Design review of the part built by this model. Coordinates are the model's own, in mm. A direction names the side the tool comes from. Coordinates: 2 decimals unless noted, no trailing zeros. Loops run counter-clockwise (first coordinate to the right, second up) from the corner with the lowest first, then second, coordinate; pieces in that order, holes last. Notation, with made-up numbers: M -9,2 L 33,2 A16 ccw 33,8 Z; hole C -31.5,68 d1. An arc over 180 degrees is marked long. One line per item, written item: value.
```python
from build123d import *

# Parameters (mm, degrees)
EXTRUDE_1_DEPTH     = 14
SKETCH_3_R          = 4.25
CUT_EXTRUDE_1_DEPTH = 51.5
SKETCH_4_R          = 8
CUT_EXTRUDE_2_DEPTH = 46


with BuildPart() as part:
    # 草图1 → 凸台-拉伸1 (new body, symmetric)
    with BuildSketch(Plane.XY):
        Polygon((-100.5, -42.991652571), (-79.5, -42.991652571), (-79.5, 0.008347429), (79.5, 0.008347429), (79.5, -42.991652571), (100.5, -42.991652571), (100.5, -23.151157314), (81.63217636, 7.508347429), (-81.63217636, 7.508347429), (-100.5, -23.151157314), align=None)
    extrude(amount=EXTRUDE_1_DEPTH, both=True)

    # 草图3 → 切除-拉伸1 (cut, through all)
    with BuildSketch(Plane.XZ.offset(42.991652571)):
        with Locations((-90, 0)):
            Circle(SKETCH_3_R)
        with Locations((90, 0)):
            Circle(SKETCH_3_R)
    extrude(amount=-CUT_EXTRUDE_1_DEPTH, mode=Mode.SUBTRACT)

    # 草图4 → 切除-拉伸2 (cut)
    with BuildSketch(Plane(origin=(0, 7.508347429, 0), x_dir=(1, 0, 0), z_dir=(0, 1, 0))):
        with Locations((-90, 0)):
            Circle(SKETCH_4_R)
        with Locations((90, 0)):
            Circle(SKETCH_4_R)
    extrude(amount=-CUT_EXTRUDE_2_DEPTH, mode=Mode.SUBTRACT)


solid = part.part
```
(1) We need section C-C on x = 90. State the section outline as (y, z) points.
Reply:
outline: M -42.99,-14 L -6.09,-14 L -6.09,-8 L -38.49,-8 L -38.49,-4.25 L -42.99,-4.25 Z; M -42.99,4.25 L -38.49,4.25 L -38.49,8 L -6.09,8 L -6.09,14 L -42.99,14 Z
(2) We need section B-B on z = 0. State the section outline as (x, y) points.
Reply:
outline: M -100.5,-42.99 L -94.25,-42.99 L -94.25,-38.49 L -98,-38.49 L -98,-19.09 L -100.5,-23.15 Z; M -85.75,-42.99 L -79.5,-42.99 L -79.5,0.01 L 79.5,0.01 L 79.5,-42.99 L 85.75,-42.99 L 85.75,-38.49 L 82,-38.49 L 82,6.91 L 81.63,7.51 L -81.63,7.51 L -82,6.91 L -82,-38.49 L -85.75,-38.49 Z; M 94.25,-42.99 L 100.5,-42.99 L 100.5,-23.15 L 98,-19.09 L 98,-38.49 L 94.25,-38.49 Z
(3) Insertion check: pin 1 (7 mm diameter, centred on x = 90, z = 0, fed in from -Y); pin 2 (8.5 mm diameter, centred on x = -33.5, z = -5, fed in from -Y); pin 3 (13 mm diameter, centred on x = -89.5, z = -0.5, fed in from +Y); pin 4 (13 mm diameter, centred on x = 86, z = 1.5, fed in from +Y). Each pin has a flat end and moves straight along its axis. Give the tip position at first contact, or say it passes through.
Reply:
pin 1: passes through
pin 2: stops at y = 0.01
pin 3: stops at y = -38.49
pin 4: stops at y = 7.51
(4) We need section A-A on y = -16. State the section outline as (x, z) points.
Reply:
outline: M -96.1,-14 L -79.5,-14 L -79.5,14 L -96.1,14 L -96.1,5.18 A8 cw long -96.1,-5.18 Z; M 79.5,-14 L 96.1,-14 L 96.1,-5.18 A8 cw long 96.1,5.18 L 96.1,14 L 79.5,14 Z
(5) Mouldability with a two-part tool opening along Z and no side actions: class faces 4 (the flat face through (95.39, -14.85, 6.42)), 5 (the flat face through (7, 1, -14)), 6 (the cylindrical face through (85.754, -40.773, 0.187)), 7 (the cylindrical face through (-94.246, -40.773, 0.187)) as released by +Z, released by -Z, zero draft, split by the parting line, or undercut.
Reply:
face 4: zero draft
face 5: released by -Z
face 6: undercut
face 7: undercut
(6) We need section D-D on x = 61. State the section outline as (y, z) points, then the cut area to 3 significant figures.
Reply:
outline: M 0.01,-14 L 7.51,-14 L 7.51,14 L 0.01,14 Z
area: 210 mm2
(7) To check wall thickness, follow line 1 along X through (y, z) = (-26, 0); line 2 along X through (y, z) = (-24, -11.75); line 3 along X through (y, z) = (-26, -1.25). State the ranges of each line that lie inside material, in increasing order. Write a range as [from, to].
Reply:
line 1: x = [-100.5, -98], [-82, -79.5], [79.5, 82], [98, 100.5]
line 2: x = [-100.5, -79.5], [79.5, 100.5]
line 3: x = [-100.5, -97.9], [-82.1, -79.5], [79.5, 82.1], [97.9, 100.5]
(8) Tool access review of faces 1 (the flat face through (100.5, -33, 0)), 2 (the flat face through (-86.6, -38.492, 3.4)), 3 (the flat face through (-79.5, -22, 0)): name each direction out of +Z, -Z, +X, -X, +Y, -Y from which nothing blocks a thin tool from reaching the whole face with its end or side.
Reply:
face 1: +Z, -Z, +X, +Y, -Y
face 2: +Y
face 3: +Z, -Z, -Y
